Source: CAD feature listing. Evaluate the final solid. Frame: model axes, mm. Face numbers are marked on the shaded views. A direction names the side the tool comes from. Give positions to 0.01 mm unless a question says otherwise; leave off trailing zeros. Loops run counter-clockwise (first coordinate to the right, second up) from the corner with the lowest first, then second, coordinate; pieces in that order, holes last. Notation, with made-up numbers: M -22.75,-22 L -11.75,-22 A22 cw -11.75,6 Z; hole C -8,-3.75 d4. An arc over 180 degrees is marked long. Write item = value, one per line.
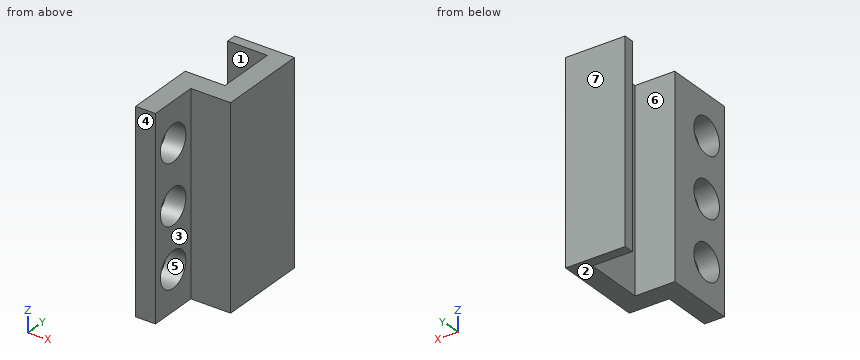
from build123d import *

# Parameters (mm, degrees)
F1_DEPTH = 20
F2_R     = 1.8
F3_DEPTH = 25


with BuildPart() as f1:
    # F0 (on Top) → F1 (new body)
    with BuildSketch(Plane.XY):
        Polygon((7.329645, -10.194992), (7.329645, -1.194992), (1.329645, -1.194992), (1.329645, -2.194992), (5.329645, -2.194992), (5.329645, -8.194992), (1.329645, -8.194992), (1.329645, -15.194992), (3.329645, -15.194992), (3.329645, -10.194992), align=None)
    extrude(amount=F1_DEPTH)

    # F2 (on face) → F3 (cut)
    with BuildSketch(Plane.YZ.offset(3.329645)):
        with Locations((-12.694992, 16)):
            Circle(F2_R)
        with Locations((-12.694992, 10)):
            Circle(F2_R)
        with Locations((-12.694992, 4)):
            Circle(F2_R)
    extrude(amount=-F3_DEPTH, mode=Mode.SUBTRACT)


solid = f1.part
1. Cut plane A-A, the plane x = 2.5. Return the cut outline in (y, z) (3 decimals), then the cut area to 3 significant figures.
Derived:
outline = M -15.195,0 L -8.195,0 L -8.195,20 L -15.195,20 Z; M -2.195,0 L -1.195,0 L -1.195,20 L -2.195,20 Z; hole C -12.695,4 d3.6; hole C -12.695,10 d3.6; hole C -12.695,16 d3.6
area = 129 mm²
2. Cut plane B-B, the plane z = 10. Return the cut outline in (x, y) (3 decimals).
Derived:
outline = M 1.33,-15.195 L 3.33,-15.195 L 3.33,-14.495 L 1.33,-14.495 Z; M 1.33,-10.895 L 3.33,-10.895 L 3.33,-10.195 L 7.33,-10.195 L 7.33,-1.195 L 1.33,-1.195 L 1.33,-2.195 L 5.33,-2.195 L 5.33,-8.195 L 1.33,-8.195 Z
3. Cut plane C-C, the plane z = 6.25. Return the cut outline in (x, y) (3 decimals).
Derived:
outline = M 1.33,-15.195 L 3.33,-15.195 L 3.33,-10.195 L 7.33,-10.195 L 7.33,-1.195 L 1.33,-1.195 L 1.33,-2.195 L 5.33,-2.195 L 5.33,-8.195 L 1.33,-8.195 Z
4. First-contact query: pin 1 Ø1 at (y, z) = (-3, 2.5) entering from -X; pin 2 Ø5.5 at (y, z) = (-13.5, 13) entering from +X; pin 3 Ø1 at (x, z) = (4, 6) entering from -Y (3 decimals). Flat tips, straight axial feed; report the tip coordinate or a pass-through.
Derived:
pin_1 = 5.33
pin_2 = 3.33
pin_3 = -10.195
5. Material intervals for probe 1 along Y at (x, z) = (3.75, 17) (3 decimals); probe 2 along Y at (x, z) = (1.7, 1.5) (3 decimals); probe 3 along Y at (x, z) = (2.35, 8.75) (3 decimals), sorted ascending. Write a range as from..to.
Derived:
probe_1 = -10.195..-8.195, -2.195..-1.195
probe_2 = -15.195..-8.195, -2.195..-1.195
probe_3 = -15.195..-13.99, -11.4..-8.195, -2.195..-1.195
6. Pull-direction query (Y, two-part tool) for the marked faces 4, 5, 6 and 7; classes: +Y half, -Y half, draft (parallel to the pull), parting line (faces both ways), or undercut.
Derived:
face_4 = -Y half
face_5 = undercut
face_6 = undercut
face_7 = +Y half
7. Reachability of the marked faces 1, 2 and 3 from +Z, -Z, +X, -X, +Y, -Y: full face, straight path, thin tool, end or side. Return the list, or none.
Derived:
face_1 = +Z, -Z, -X
face_2 = -Z, +X, -X, +Y, -Y
face_3 = +Z, -Z, +X, -Y
8. Cut plane D-D, the plane y = -6. Return the cut outline in (x, z).
Derived:
outline = M 5.33,0 L 7.33,0 L 7.33,20 L 5.33,20 Z
